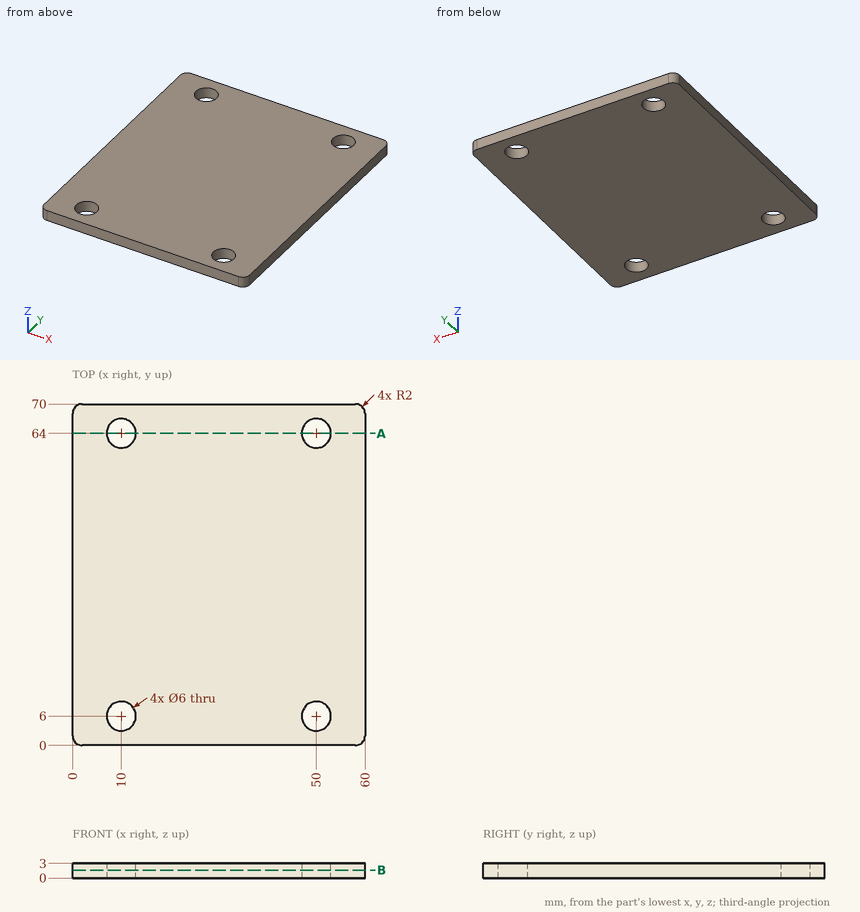
For this review, use the dimensioned drawing (mm, ordinates from the lowest corner) and the shaded views. Coordinates: 2 decimals unless noted, no trailing zeros. Write each loop counter-clockwise with the first axis right and the second up, starting at its lowest first coordinate (ties: lowest second). Pieces come first, ordered by that corner, then holes. Notation, with made-up numbers: (76, 19.25) - (119, 19.25) arc R17 ccw to (119, 30.25) - close; hole circle Ø11 at (79.5, -12). An arc over 180 degrees is marked (long way). Answer as a JSON object with one key per item and string values. Group by question number.
1. Clearance check with flat-ended pins moving along their axes: pin 1 Ø3 at (x, y) = (49.5, 50) entering from -Z; pin 2 Ø5.5 at (x, y) = (50, 64) entering from +Z. State where each tip first meets the part, or that it passes through.
2. Add section B-B (z = 1.6). Give the boundary of the cut face in (x, y).
3. To check wall thickness, follow probe 1 along Y at (x, z) = (50, 1.65); probe 2 along X at (y, z) = (63, 0.25); probe 3 along Y at (x, z) = (7.5, 1.9). State the ranges of each line that lie inside material, in increasing order.
4. Add section A-A (y = 64). Give the boundary of the cut face in (x, z), plus the area to 3 significant figures.
Findings:
{
 "1": {"pin 1": "z = 0", "pin 2": "through"},
 "2": {"outline": "(0, 2) arc R2 ccw to (2, 0) - (58, 0) arc R2 ccw to (60, 2) - (60, 68) arc R2 ccw to (58, 70) - (2, 70) arc R2 ccw to (0, 68) - close; hole circle Ø6 at (10, 6); hole circle Ø6 at (10, 64); hole circle Ø6 at (50, 6); hole circle Ø6 at (50, 64)"},
 "3": {"probe 1": "0 to 3, 9 to 61, 67 to 70", "probe 2": "0 to 7.17, 12.83 to 47.17, 52.83 to 60", "probe 3": "0 to 4.34, 7.66 to 62.34, 65.66 to 70"},
 "4": {"outline": "(0, 0) - (7, 0) - (7, 3) - (0, 3) - close; (13, 0) - (47, 0) - (47, 3) - (13, 3) - close; (53, 0) - (60, 0) - (60, 3) - (53, 3) - close", "area": "144 mm²"}
}
